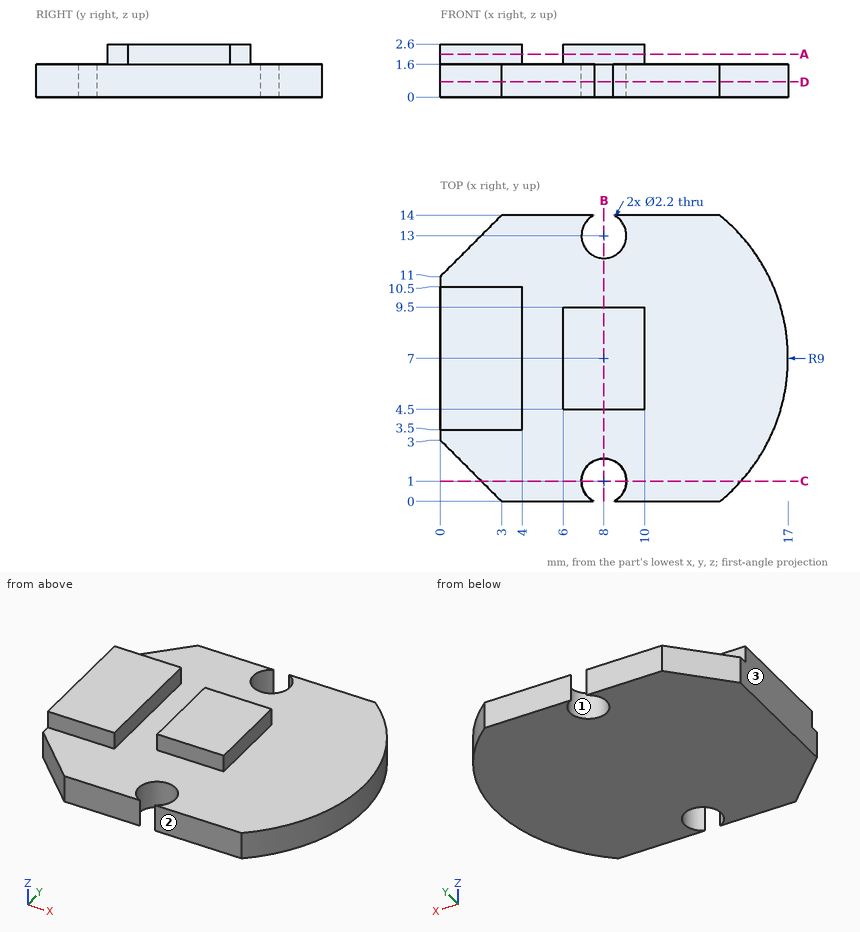
The drawing under review shows one solid part. Ordinate dimensions are in mm from its lowest x, y, z. Round coordinates to 2 decimals unless told otherwise and drop trailing zeros. Write each loop counter-clockwise with the first axis right and the second up, starting at its lowest first coordinate (ties: lowest second). Pieces come first, ordered by that corner, then holes. Notation, with made-up numbers: (58, 48) - (117, 48) arc R28 cw to (117, 83) - close; hole circle Ø1 at (1, 7.25). An arc over 180 degrees is marked (long way). Write each question's results on one line, items separated by ' | '.
Item 1: Take a section at A-A on z = 2.1. State the section outline as (x, y) points, then the cut area to 3 significant figures.
Calculated:
outline: (0, 3.5) - (4, 3.5) - (4, 10.5) - (0, 10.5) - close; (6, 4.5) - (10, 4.5) - (10, 9.5) - (6, 9.5) - close | area: 48.0 mm^2
Item 2: For pin 1 (0.8 mm diameter, centred on x = 8, z = 2.5, fed in from -Y); pin 2 (1.5 mm diameter, centred on x = 2, y = 1.5, fed in from +Z); pin 3 (0.5 mm diameter, centred on y = 6, z = 2, fed in from +X), all flat-tipped, find the tip position at first contact; note any pin that passes through.
Calculated:
pin 1: stops at y = 4.5 | pin 2: stops at z = 1.6 | pin 3: stops at x = 10
Item 3: Take a section at D-D on z = 0.75. State the section outline as (x, y) points, then the cut area to 3 significant figures.
Calculated:
outline: (0, 3) - (3, 0) - (7.54, 0) arc R1.1 cw (long way) to (8.46, 0) - (13.66, 0) arc R9 ccw to (13.66, 14) - (8.46, 14) arc R1.1 cw (long way) to (7.54, 14) - (3, 14) - (0, 11) - close | area: 207 mm^2
Item 4: Take a section at C-C on y = 1. State the section outline as (x, z) points.
Calculated:
outline: (2, 0) - (6.9, 0) - (6.9, 1.6) - (2, 1.6) - close; (9.1, 0) - (14.71, 0) - (14.71, 1.6) - (9.1, 1.6) - close
Item 5: Draft analysis for pull direction Y (two halves, no side actions). For the marked faces 1, 2 and 3, state which applies: pulls with the +Y half, pulls with the -Y half, needs draft (parallel to the pull), parting line crosses it, or undercut.
Calculated:
face 1: undercut | face 2: pulls with the -Y half | face 3: needs draft
Item 6: To check wall thickness, follow line 1 along X through (y, z) = (9, 2.1); line 2 along Z through (x, y) = (10.25, 3.75); line 3 along Y through (x, z) = (8, 1.1). State the ranges of each line that lie inside material, in increasing order. Write a range as from..to.
Calculated:
line 1: x = 0..4, 6..10 | line 2: z = 0..1.6 | line 3: y = 2.1..11.9
Item 7: Take a section at B-B on x = 8. State the section outline as (y, z) points.
Calculated:
outline: (2.1, 0) - (11.9, 0) - (11.9, 1.6) - (9.5, 1.6) - (9.5, 2.6) - (4.5, 2.6) - (4.5, 1.6) - (2.1, 1.6) - close
